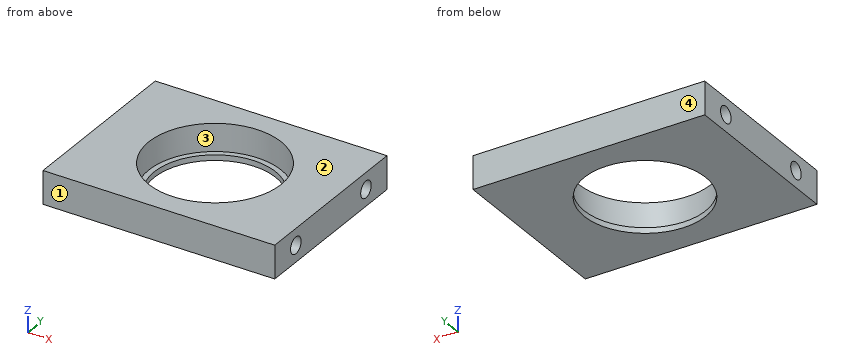
```python
from build123d import *

# Parameters (mm, degrees)
SKETCH_1_W                = 42
SKETCH_1_H                = 32
EXTRUDE_1_DEPTH           = 6
HOLE_WIZARD_3_0_3_1_D     = 3
HOLE_WIZARD_3_0_3_1_DEPTH = 6
HOLE_WIZARD_3_0_3_2_D     = 3
HOLE_WIZARD_3_0_3_2_DEPTH = 6
M24X2_0_1_D               = 22
M24X2_0_1_CBORE_D         = 24
M24X2_0_1_CBORE_DEPTH     = 4
SKETCH_8_R                = 12
CUT_EXTRUDE_1_DEPTH       = 5


with BuildPart() as part:
    # 草图1 → 凸台-拉伸1 (new body)
    with BuildSketch(Plane.XY.offset(6)):
        Rectangle(SKETCH_1_W, SKETCH_1_H)
    extrude(amount=-EXTRUDE_1_DEPTH)

    # Ø3.0 (3) 直径孔1
    with Locations(Plane(origin=(21, 0, 0), x_dir=(0, 0, -1), z_dir=(1, 0, 0))):
        with Locations((-3, -10), (-3, 10)):
            Hole(HOLE_WIZARD_3_0_3_1_D / 2, depth=HOLE_WIZARD_3_0_3_1_DEPTH)

    # Ø3.0 (3) 直径孔2
    with Locations(Plane.ZY.offset(21)):
        with Locations((3, -10), (3, 10)):
            Hole(HOLE_WIZARD_3_0_3_2_D / 2, depth=HOLE_WIZARD_3_0_3_2_DEPTH)

    # M24x2.0 螺纹孔1 (through all)
    with Locations(Plane.XY.offset(6)):
        with Locations((0, 0)):
            CounterBoreHole(M24X2_0_1_D / 2, M24X2_0_1_CBORE_D / 2, M24X2_0_1_CBORE_DEPTH)

    # 草图8 → 切除-拉伸1 (cut)
    with BuildSketch(Plane.XY.offset(6)):
        Circle(SKETCH_8_R)
    extrude(amount=-CUT_EXTRUDE_1_DEPTH, mode=Mode.SUBTRACT)


solid = part.part
```
For this review, take the finished solid that the model builds, in its own axes (mm). Face numbers are marked on the shaded views. Coordinates: 2 decimals unless noted, no trailing zeros. Write each loop counter-clockwise with the first axis right and the second up, starting at its lowest first coordinate (ties: lowest second). Pieces come first, ordered by that corner, then holes.
(1) Add section C-C on y = 0. Give the boundary of the cut face in (x, z), then the cut area to 3 significant figures.
(2) Add section B-B on z = 3. Give the boundary of the cut face in (x, y), then the cut area to 3 significant figures.
(3) Add section A-A on x = 0. Give the boundary of the cut face in (y, z), then the cut area to 3 significant figures.
(4) Add section D-D on x = -17. Give the boundary of the cut face in (y, z).
(5) The part is to be moulded in two halves that separate along Y. For the marked faces 1, 2, 3 and 4, say which applies: +Y half, -Y half, draft (parallel to the pull), parting line (faces both ways), or undercut.
(6) Wall thickness on probe 1 along Y at (x, z) = (17.5, 2.45); probe 2 along Y at (x, z) = (0, 0.35); probe 3 along Y at (x, z) = (-17.5, 4.05): over which ranges is each line inside the solid? List them lowest first.
(7) For pin 1 Ø1.8 at (y, z) = (10, 3) entering from -X; pin 2 Ø3.5 at (y, z) = (9.5, 3.5) entering from +X; pin 3 Ø7 at (x, y) = (2, 5.5) entering from +Z, all flat-tipped, find the tip position at first contact; note any pin that passes through.
Answer sheet:
1. outline: (-21, 0) - (-11, 0) - (-11, 1) - (-12, 1) - (-12, 6) - (-21, 6) - close; (11, 0) - (21, 0) - (21, 6) - (12, 6) - (12, 1) - (11, 1) - close
1. area: 110 mm2
2. outline: (-21, -16) - (21, -16) - (21, -11.5) - (15, -11.5) - (15, -8.5) - (21, -8.5) - (21, 8.5) - (15, 8.5) - (15, 11.5) - (21, 11.5) - (21, 16) - (-21, 16) - (-21, 11.5) - (-15, 11.5) - (-15, 8.5) - (-21, 8.5) - (-21, -8.5) - (-15, -8.5) - (-15, -11.5) - (-21, -11.5) - close; hole circle Ø24 at (0, 0)
2. area: 820 mm2
3. outline: (-16, 0) - (-11, 0) - (-11, 1) - (-12, 1) - (-12, 6) - (-16, 6) - close; (11, 0) - (16, 0) - (16, 6) - (12, 6) - (12, 1) - (11, 1) - close
3. area: 50.0 mm2
4. outline: (-16, 0) - (16, 0) - (16, 6) - (-16, 6) - close; hole circle Ø3 at (-10, 3); hole circle Ø3 at (10, 3)
5. face 1: -Y half
5. face 2: draft
5. face 3: undercut
5. face 4: +Y half
6. probe 1: y = -16 to -11.4, -8.6 to 8.6, 11.4 to 16
6. probe 2: y = -16 to -11, 11 to 16
6. probe 3: y = -16 to -11.07, -8.93 to 8.93, 11.07 to 16
7. pin 1: stops at x = -15
7. pin 2: stops at x = 21
7. pin 3: passes through
